Part model, mm, in its own coordinate system. Face numbers are marked on the shaded views. Round coordinates to 2 decimals unless told otherwise and drop trailing zeros. Write each loop counter-clockwise with the first axis right and the second up, starting at its lowest first coordinate (ties: lowest second). Pieces come first, ordered by that corner, then holes.
1) Saw through at D-D on z = 12. Count the separate pieces of the cut face and the enclosed holes in it, and give its area (3 significant figures).
2) Flat gauge pins, fed straight in: pin 1 (0.9 mm diameter, centred on y = 3, z = 51.5, fed in from -X); pin 2 (2 mm diameter, centred on x = 168.5, y = 4.5, fed in from +Z); pin 3 (1.4 mm diameter, centred on x = 185, y = 6, fed in from -Z). Where does each tip first touch, or does it go through?
3) Saw through at A-A on x = 193.5. Write the cut outline in (y, z), and give its area (3 significant figures).
4) Saw through at C-C on z = 30. Write the cut outline in (x, y).
5) Pull direction X, two halves, no side cores. Call the marked faces 1 and 2: +X half, -X half, draft (parallel to the pull), parting line (faces both ways), or undercut.
6) Drill centre lines: L1, parallel to Z at x = 179.5, y = 4; L2, parallel to X at y = 0.75, z = 6; L3, parallel to X at y = 0.3, z = 34. Where is each one in solid material? Low to high.
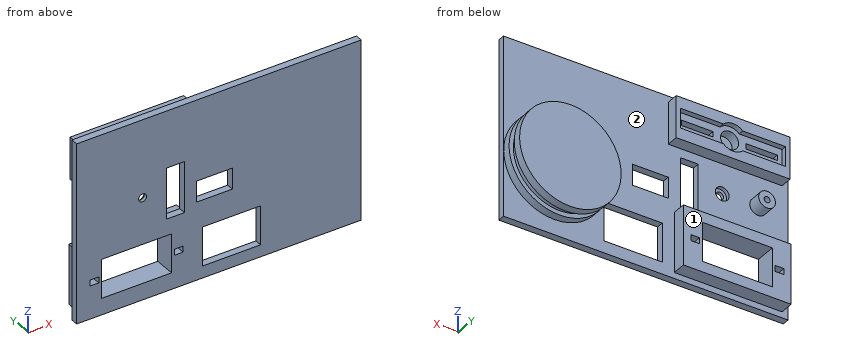
```python
from build123d import *

# Parameters (mm, degrees)
SKETCH1_W            = 95
SKETCH1_H            = 2.4
BOSS_EXTRUDE1_DEPTH  = 60
BOSS_EXTRUDE2_START  = 2
SKETCH2_W            = 36
SKETCH2_H            = 4.6
BOSS_EXTRUDE2_DEPTH  = 20
BOSS_EXTRUDE3_START  = 5.5
SKETCH3_W            = 23.4
SKETCH3_H            = 9
BOSS_EXTRUDE3_DEPTH  = 13
BOSS_EXTRUDE4_START  = 11
SKETCH4_W            = 2.9
SKETCH4_H            = 9
BOSS_EXTRUDE4_DEPTH  = 2
BOSS_EXTRUDE5_START  = 11
SKETCH5_W            = 2.9
SKETCH5_H            = 9
BOSS_EXTRUDE5_DEPTH  = 2
BOSS_EXTRUDE6_START  = 4
SKETCH6_W            = 19.4
SKETCH6_H            = 4.4
BOSS_EXTRUDE6_DEPTH  = 13
BOSS_EXTRUDE7_START  = 2.4
SKETCH7_R            = 2.8
BOSS_EXTRUDE7_DEPTH  = 4.5
BOSS_EXTRUDE8_START  = 1.6
SKETCH8_R            = 1
BOSS_EXTRUDE8_DEPTH  = 6.3
BOSS_EXTRUDE9_START  = -1
SKETCH9_R            = 1.3
BOSS_EXTRUDE9_DEPTH  = 4.4
BOSS_EXTRUDE10_START = 1.1
SKETCH10_R           = 2.3
BOSS_EXTRUDE10_DEPTH = 2.3
BOSS_EXTRUDE11_START = 24
SKETCH11_W           = 6
SKETCH11_H           = 4.4
BOSS_EXTRUDE11_DEPTH = 17
BOSS_EXTRUDE12_START = 26
SKETCH12_W           = 12
SKETCH12_H           = 4.4
BOSS_EXTRUDE12_DEPTH = 7
BOSS_EXTRUDE13_START = 2.4
SKETCH13_R           = 16.95
BOSS_EXTRUDE13_DEPTH = 8
BOSS_EXTRUDE14_START = 5.1
SKETCH14_R           = 20
BOSS_EXTRUDE14_DEPTH = 2.6
BOSS_EXTRUDE15_START = 5.1
SKETCH15_R           = 15.5
BOSS_EXTRUDE15_DEPTH = 2.6
BOSS_EXTRUDE16_START = 44
SKETCH16_W           = 38
SKETCH16_H           = 4
BOSS_EXTRUDE16_DEPTH = 14
BOSS_EXTRUDE17_START = 4.6
SKETCH17_R           = 4.6
BOSS_EXTRUDE17_DEPTH = 2.3
BOSS_EXTRUDE18_START = 47.7
SKETCH18_W           = 17.5
SKETCH18_H           = 2.3
BOSS_EXTRUDE18_DEPTH = 6.6
BOSS_EXTRUDE19_START = 50.1
SKETCH19_W           = 10.5
SKETCH19_H           = 6
BOSS_EXTRUDE19_DEPTH = 1.8
BOSS_EXTRUDE20_START = 47.7
SKETCH20_W           = 17.5
SKETCH20_H           = 2.3
BOSS_EXTRUDE20_DEPTH = 6.6
BOSS_EXTRUDE21_START = 50.1
SKETCH21_W           = 10.5
SKETCH21_H           = 6
BOSS_EXTRUDE21_DEPTH = 1.8
BOSS_EXTRUDE22_START = 1.4
SKETCH22_R           = 3
BOSS_EXTRUDE22_DEPTH = 6


with BuildPart() as part:
    # Sketch1 → Boss-Extrude1 (new body)
    with BuildSketch(Plane.XY):
        with Locations((197.5, 1.2)):
            Rectangle(SKETCH1_W, SKETCH1_H)
    extrude(amount=BOSS_EXTRUDE1_DEPTH)

    # Sketch2 → Boss-Extrude2 (add)
    with BuildSketch(Plane.XY.offset(BOSS_EXTRUDE2_START)):
        with Locations((170, 4.7)):
            Rectangle(SKETCH2_W, SKETCH2_H)
    extrude(amount=BOSS_EXTRUDE2_DEPTH)


with BuildPart() as body_2:
    # Sketch3 → Boss-Extrude3 (new body)
    with BuildSketch(Plane.XY.offset(BOSS_EXTRUDE3_START)):
        with Locations((170, 3.5)):
            Rectangle(SKETCH3_W, SKETCH3_H)
    extrude(amount=BOSS_EXTRUDE3_DEPTH)


with BuildPart() as part_1:
    add(part.part)

    # Combine1: cut body 2
    add(body_2.part, mode=Mode.SUBTRACT)


with BuildPart() as body_2_2:
    # Sketch4 → Boss-Extrude4 (new body)
    with BuildSketch(Plane.XY.offset(BOSS_EXTRUDE4_START)):
        with Locations((155.925, 3.5)):
            Rectangle(SKETCH4_W, SKETCH4_H)
    extrude(amount=BOSS_EXTRUDE4_DEPTH)


with BuildPart() as part_2:
    add(part_1.part)

    # Combine2: cut body 2 2
    add(body_2_2.part, mode=Mode.SUBTRACT)


with BuildPart() as body_2_3:
    # Sketch5 → Boss-Extrude5 (new body)
    with BuildSketch(Plane.XY.offset(BOSS_EXTRUDE5_START)):
        with Locations((184.075, 3.5)):
            Rectangle(SKETCH5_W, SKETCH5_H)
    extrude(amount=BOSS_EXTRUDE5_DEPTH)


with BuildPart() as part_3:
    add(part_2.part)

    # Combine3: cut body 2 3
    add(body_2_3.part, mode=Mode.SUBTRACT)


with BuildPart() as body_2_4:
    # Sketch6 → Boss-Extrude6 (new body)
    with BuildSketch(Plane.XY.offset(BOSS_EXTRUDE6_START)):
        with Locations((201.7, 1.2)):
            Rectangle(SKETCH6_W, SKETCH6_H)
    extrude(amount=BOSS_EXTRUDE6_DEPTH)


with BuildPart() as part_4:
    add(part_3.part)

    # Combine4: cut body 2 4
    add(body_2_4.part, mode=Mode.SUBTRACT)

    # Sketch7 → Boss-Extrude7 (add)
    with BuildSketch(Plane(origin=(0, 0, 0), x_dir=(1, 0, 0), z_dir=(0, 1, 0)).offset(BOSS_EXTRUDE7_START)):
        with Locations(Location((160, -34, 0), (0, 0, 90))):
            Circle(SKETCH7_R)
    extrude(amount=BOSS_EXTRUDE7_DEPTH)


with BuildPart() as body_2_5:
    # Sketch8 → Boss-Extrude8 (new body)
    with BuildSketch(Plane(origin=(0, 0, 0), x_dir=(1, 0, 0), z_dir=(0, 1, 0)).offset(BOSS_EXTRUDE8_START)):
        with Locations(Location((160, -34, 0), (0, 0, 270))):
            Circle(SKETCH8_R)
    extrude(amount=BOSS_EXTRUDE8_DEPTH)


with BuildPart() as part_5:
    add(part_4.part)

    # Combine5: cut body 2 5
    add(body_2_5.part, mode=Mode.SUBTRACT)


with BuildPart() as body_2_6:
    # Sketch9 → Boss-Extrude9 (new body)
    with BuildSketch(Plane(origin=(0, 0, 0), x_dir=(1, 0, 0), z_dir=(0, 1, 0)).offset(BOSS_EXTRUDE9_START)):
        with Locations(Location((172, -34, 0), (0, 0, 270))):
            Circle(SKETCH9_R)
    extrude(amount=BOSS_EXTRUDE9_DEPTH)


with BuildPart() as part_6:
    add(part_5.part)

    # Combine6: cut body 2 6
    add(body_2_6.part, mode=Mode.SUBTRACT)


with BuildPart() as body_2_7:
    # Sketch10 → Boss-Extrude10 (new body)
    with BuildSketch(Plane(origin=(0, 0, 0), x_dir=(1, 0, 0), z_dir=(0, 1, 0)).offset(BOSS_EXTRUDE10_START)):
        with Locations(Location((172, -34, 0), (0, 0, 270))):
            Circle(SKETCH10_R)
    extrude(amount=BOSS_EXTRUDE10_DEPTH)


with BuildPart() as part_7:
    add(part_6.part)

    # Combine7: cut body 2 7
    add(body_2_7.part, mode=Mode.SUBTRACT)


with BuildPart() as body_2_8:
    # Sketch11 → Boss-Extrude11 (new body)
    with BuildSketch(Plane.XY.offset(BOSS_EXTRUDE11_START)):
        with Locations((183, 1.2)):
            Rectangle(SKETCH11_W, SKETCH11_H)
    extrude(amount=BOSS_EXTRUDE11_DEPTH)


with BuildPart() as part_8:
    add(part_7.part)

    # Combine8: cut body 2 8
    add(body_2_8.part, mode=Mode.SUBTRACT)


with BuildPart() as body_2_9:
    # Sketch12 → Boss-Extrude12 (new body)
    with BuildSketch(Plane.XY.offset(BOSS_EXTRUDE12_START)):
        with Locations((196, 1.2)):
            Rectangle(SKETCH12_W, SKETCH12_H)
    extrude(amount=BOSS_EXTRUDE12_DEPTH)


with BuildPart() as part_9:
    add(part_8.part)

    # Combine9: cut body 2 9
    add(body_2_9.part, mode=Mode.SUBTRACT)

    # Sketch13 → Boss-Extrude13 (add)
    with BuildSketch(Plane(origin=(0, 0, 0), x_dir=(1, 0, 0), z_dir=(0, 1, 0)).offset(BOSS_EXTRUDE13_START)):
        with Locations(Location((228, -22, 0), (0, 0, 90))):
            Circle(SKETCH13_R)
    extrude(amount=BOSS_EXTRUDE13_DEPTH)


with BuildPart() as body_2_10:
    # Sketch14 → Boss-Extrude14 (new body)
    with BuildSketch(Plane(origin=(0, 0, 0), x_dir=(1, 0, 0), z_dir=(0, 1, 0)).offset(BOSS_EXTRUDE14_START)):
        with Locations(Location((228, -22, 0), (0, 0, 270))):
            Circle(SKETCH14_R)
    extrude(amount=BOSS_EXTRUDE14_DEPTH)


with BuildPart() as part_10:
    add(part_9.part)

    # Combine10: cut body 2 10
    add(body_2_10.part, mode=Mode.SUBTRACT)

    # Sketch15 → Boss-Extrude15 (add)
    with BuildSketch(Plane(origin=(0, 0, 0), x_dir=(1, 0, 0), z_dir=(0, 1, 0)).offset(BOSS_EXTRUDE15_START)):
        with Locations(Location((228, -22, 0), (0, 0, 270))):
            Circle(SKETCH15_R)
    extrude(amount=BOSS_EXTRUDE15_DEPTH)

    # Sketch16 → Boss-Extrude16 (add)
    with BuildSketch(Plane.XY.offset(BOSS_EXTRUDE16_START)):
        with Locations((171, 4.4)):
            Rectangle(SKETCH16_W, SKETCH16_H)
    extrude(amount=BOSS_EXTRUDE16_DEPTH)


with BuildPart() as body_2_11:
    # Sketch17 → Boss-Extrude17 (new body)
    with BuildSketch(Plane(origin=(0, 0, 0), x_dir=(1, 0, 0), z_dir=(0, 1, 0)).offset(BOSS_EXTRUDE17_START)):
        with Locations(Location((171, -51, 0), (0, 0, 270))):
            Circle(SKETCH17_R)
    extrude(amount=BOSS_EXTRUDE17_DEPTH)


with BuildPart() as part_11:
    add(part_10.part)

    # Combine11: cut body 2 11
    add(body_2_11.part, mode=Mode.SUBTRACT)


with BuildPart() as body_2_12:
    # Sketch18 → Boss-Extrude18 (new body)
    with BuildSketch(Plane.XY.offset(BOSS_EXTRUDE18_START)):
        with Locations((179.75, 5.75)):
            Rectangle(SKETCH18_W, SKETCH18_H)
    extrude(amount=BOSS_EXTRUDE18_DEPTH)


with BuildPart() as part_12:
    add(part_11.part)

    # Combine12: cut body 2 12
    add(body_2_12.part, mode=Mode.SUBTRACT)


with BuildPart() as body_2_13:
    # Sketch19 → Boss-Extrude19 (new body)
    with BuildSketch(Plane.XY.offset(BOSS_EXTRUDE19_START)):
        with Locations((181.75, 4.4)):
            Rectangle(SKETCH19_W, SKETCH19_H)
    extrude(amount=BOSS_EXTRUDE19_DEPTH)


with BuildPart() as part_13:
    add(part_12.part)

    # Combine13: cut body 2 13
    add(body_2_13.part, mode=Mode.SUBTRACT)


with BuildPart() as body_2_14:
    # Sketch20 → Boss-Extrude20 (new body)
    with BuildSketch(Plane.XY.offset(BOSS_EXTRUDE20_START)):
        with Locations((162.25, 5.75)):
            Rectangle(SKETCH20_W, SKETCH20_H)
    extrude(amount=BOSS_EXTRUDE20_DEPTH)


with BuildPart() as part_14:
    add(part_13.part)

    # Combine14: cut body 2 14
    add(body_2_14.part, mode=Mode.SUBTRACT)


with BuildPart() as body_2_15:
    # Sketch21 → Boss-Extrude21 (new body)
    with BuildSketch(Plane.XY.offset(BOSS_EXTRUDE21_START)):
        with Locations((160.25, 4.4)):
            Rectangle(SKETCH21_W, SKETCH21_H)
    extrude(amount=BOSS_EXTRUDE21_DEPTH)


with BuildPart() as part_15:
    add(part_14.part)

    # Combine15: cut body 2 15
    add(body_2_15.part, mode=Mode.SUBTRACT)


with BuildPart() as body_2_16:
    # Sketch22 → Boss-Extrude22 (new body)
    with BuildSketch(Plane(origin=(0, 0, 0), x_dir=(1, 0, 0), z_dir=(0, 1, 0)).offset(BOSS_EXTRUDE22_START)):
        with Locations(Location((171, -51, 0), (0, 0, 270))):
            Circle(SKETCH22_R)
    extrude(amount=BOSS_EXTRUDE22_DEPTH)


with BuildPart() as part_16:
    add(part_15.part)

    # Combine16: cut body 2 16
    add(body_2_16.part, mode=Mode.SUBTRACT)


solid = part_16.part
```
Completed:
1. separate pieces: 5
1. enclosed holes: 0
1. area: 352 mm2
2. pin 1: stops at x = 152
2. pin 2: stops at z = 58
2. pin 3: stops at z = 2
3. outline: (0, 0) - (2.4, 0) - (2.4, 4) - (0, 4) - close; (0, 17) - (2.4, 17) - (2.4, 26) - (0, 26) - close; (0, 33) - (2.4, 33) - (2.4, 60) - (0, 60) - close
3. area: 96.0 mm2
4. outline: (150, 0) - (180, 0) - (180, 2.4) - (150, 2.4) - close; (186, 0) - (190, 0) - (190, 2.4) - (186, 2.4) - close; (202, 0) - (245, 0) - (245, 2.4) - (242.94, 2.4) - (242.94, 5.1) - (241.28, 5.1) - (241.28, 7.7) - (242.94, 7.7) - (242.94, 10.4) - (213.06, 10.4) - (213.06, 7.7) - (214.72, 7.7) - (214.72, 5.1) - (213.06, 5.1) - (213.06, 2.4) - (202, 2.4) - close
5. face 1: draft
5. face 2: undercut
6. L1: z = 2 to 5.5, 18.5 to 22, 44 to 50.1, 51.9 to 58
6. L2: x = 150 to 158.3, 181.7 to 192, 211.4 to 245
6. L3: x = 150 to 170.7, 173.3 to 180, 186 to 245
